Check sheet for the modelled part. Datum: model origin and axes. Units: mm. Round coordinates to 2 decimals unless told otherwise and drop trailing zeros. Loops run counter-clockwise (first coordinate to the right, second up) from the corner with the lowest first, then second, coordinate; pieces in that order, holes last. Notation, with made-up numbers: (15.5, -8) -> (34.5, -8) arc R8 cw to (34.5, -2) -> close; hole circle Ø2 at (47.5, 53). An arc over 180 degrees is marked (long way). One line per question, with ' | ' between items.
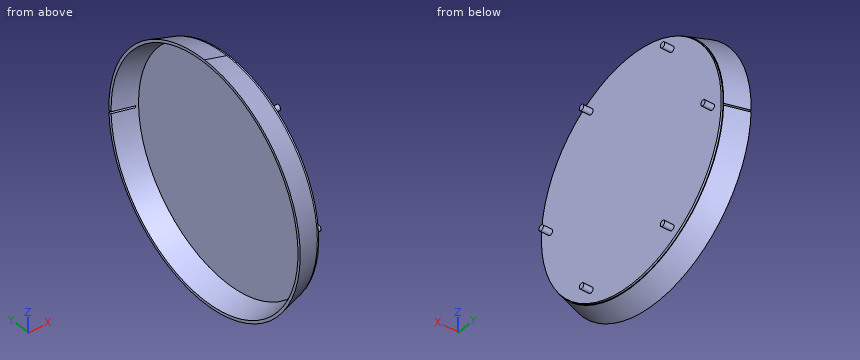
```python
from build123d import *

# Parameters (mm, degrees)
CUT_EXTRUDE1_REACH  = 94.704
SKETCH3_W           = 1
SKETCH3_H           = 9
SKETCH7_R           = 61.102685311
BOSS_EXTRUDE1_DEPTH = 1
SKETCH8_R           = 1.5
BOSS_EXTRUDE2_DEPTH = 5
CIRPATTERN1_COUNT   = 6


with BuildPart() as part:
    # Sketch2 → Revolve1 (revolve)
    with BuildSketch(Plane.XY, mode=Mode.PRIVATE) as revolve1_sk:
        Polygon((0, 65), (0, 63.5), (12, 60), (12, 61.5), align=None)
    revolve(revolve1_sk.sketch.rotate(Axis((0, 0, 0), (1, 0, 0)), 90), axis=Axis((0, 0, 0), (1, 0, 0)))

    # Cut-Extrude1: up to this face of the body (flat: up to its plane)
    cut_extrude1_end = Plane(part.part.faces().sort_by_distance((0, 0, -64.816152237))[0])
    # Sketch3 → Cut-Extrude1 (cut, up to the picked face)
    with BuildSketch(Plane(origin=(12, 0, 0), x_dir=(0, 0, -1), z_dir=(1, 0, 0)), mode=Mode.PRIVATE) as cut_extrude1_sk1:
        with Locations((1.827954501, 64.835601496)):
            Rectangle(SKETCH3_W, SKETCH3_H)
    cut_extrude1_tool1 = split(extrude(cut_extrude1_sk1.sketch, amount=-CUT_EXTRUDE1_REACH, mode=Mode.PRIVATE), bisect_by=cut_extrude1_end, keep=Keep.BOTH, mode=Mode.PRIVATE)
    add(cut_extrude1_tool1.solids().sort_by(Axis((12, 64.835601, -1.827955), (-1, 0, 0)))[0], mode=Mode.SUBTRACT)

    # Sketch7 → Boss-Extrude1 (add)
    with BuildSketch(Plane(origin=(12, 0, 0), x_dir=(0, 0, -1), z_dir=(1, 0, 0))):
        with Locations(Location((0, 0, 0), (0, 0, 88.754683549))):
            Circle(SKETCH7_R)
    extrude(amount=BOSS_EXTRUDE1_DEPTH)

    # Sketch8 → Boss-Extrude2 (add)
    with BuildSketch(Plane(origin=(13, 0, 0), x_dir=(0, 0, -1), z_dir=(1, 0, 0))):
        with Locations((0, 55)):
            Circle(SKETCH8_R)
    boss_extrude2 = extrude(amount=BOSS_EXTRUDE2_DEPTH)

    # CirPattern1: Boss-Extrude2 ×6 about axis
    cirpattern1_axis = Axis((0, 0, 0), (1, 0, 0))
    for i in range(1, CIRPATTERN1_COUNT):
        add(boss_extrude2.rotate(cirpattern1_axis, i * 360 / CIRPATTERN1_COUNT))


solid = part.part
```
(1) Scan lines: probe 1 along X at (y, z) = (39, 27); probe 2 along Y at (x, z) = (10.5, 52); probe 3 along Z at (x, y) = (4.75, -1.5). Record each from-to range of solid material in increasing order.
Answer:
probe 1: x = 12 to 13 | probe 2: y = -33.65 to -30.8, 30.8 to 33.65 | probe 3: z = -63.6 to -62.1, 62.1 to 63.6
(2) Sectioned sample at A-A, the plane x = 8.25. Record the cut outline in (y, z).
Answer:
outline: (61.05, -2.33) arc R61.09 cw (long way) to (61.08, -1.33) -> (62.58, -1.33) arc R62.59 ccw (long way) to (62.55, -2.33) -> close
(3) Go/stop test with flat-tipped pins: pin 1 (8 mm diameter, centred on x = 8.5, y = 15, fed in from -Z); pin 2 (4 mm diameter, centred on x = 7.5, z = 11.5, fed in from +Y); pin 3 (4 mm diameter, centred on x = 8.5, y = -48, fed in from -Z). Record where each tip stops, or that it passes through.
Answer:
pin 1: stops at z = -62.19 | pin 2: stops at y = 62.44 | pin 3: stops at z = -42.51
